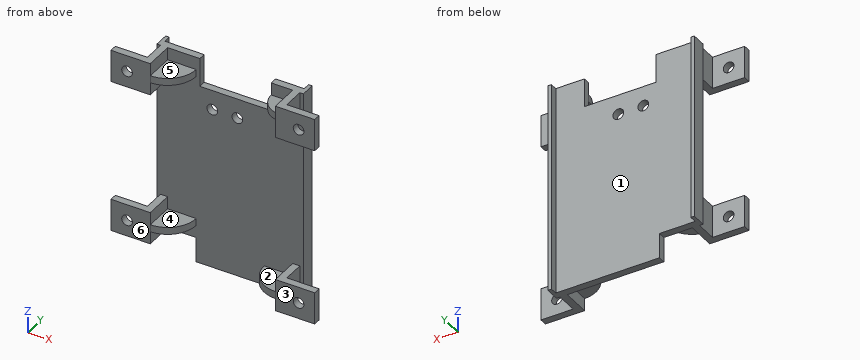
```python
from build123d import *

# Parameters (mm, degrees)
SKETCH1_W           = 57
SKETCH1_H           = 59
BOSS_EXTRUDE1_DEPTH = 10
SKETCH2_W           = 41
SKETCH2_H           = 10
CUT_EXTRUDE1_DEPTH  = 9
SKETCH4_W           = 10
SKETCH4_H           = 7
CUT_EXTRUDE3_DEPTH  = 83.643814046
SKETCH5_W           = 34
SKETCH5_H           = 10
CUT_EXTRUDE4_DEPTH  = 9
SKETCH8_W           = 20
SKETCH8_H           = 10
CUT_EXTRUDE5_DEPTH  = 8
SKETCH9_W           = 35
SKETCH9_H           = 59
CUT_EXTRUDE6_DEPTH  = 8
SKETCH10_W          = 9
SKETCH10_H          = 7
CUT_EXTRUDE7_DEPTH  = 83.643814046
SKETCH11_W          = 9
SKETCH11_H          = 9
CUT_EXTRUDE8_DEPTH  = 8
SKETCH12_W          = 9
SKETCH12_H          = 9
CUT_EXTRUDE9_DEPTH  = 8
SKETCH13_W          = 9
SKETCH13_H          = 9
CUT_EXTRUDE10_DEPTH = 8
SKETCH14_W          = 9
SKETCH14_H          = 9
CUT_EXTRUDE11_DEPTH = 8
SKETCH15_W          = 2
SKETCH15_H          = 41
CUT_EXTRUDE12_DEPTH = 8
SKETCH16_W          = 2
SKETCH16_H          = 34
CUT_EXTRUDE13_DEPTH = 8
SKETCH31_W          = 2
SKETCH31_H          = 8
REVOLVE3_ANGLE      = 90
SKETCH32_W          = 2
SKETCH32_H          = 8
REVOLVE4_ANGLE      = 90
SKETCH33_W          = 6
SKETCH33_H          = 2
REVOLVE5_ANGLE      = 90
SKETCH34_W          = 2
SKETCH34_H          = 8
REVOLVE6_ANGLE      = 90
SKETCH41_R          = 1.5
CUT_EXTRUDE14_DEPTH = 83.42572414
SKETCH42_R          = 1.5
CUT_EXTRUDE15_DEPTH = 83.643814046
SKETCH46_W          = 59
SKETCH46_H          = 2
BOSS_EXTRUDE3_DEPTH = 1
SKETCH47_W          = 1
SKETCH47_H          = 59
BOSS_EXTRUDE4_DEPTH = 2
SKETCH48_W          = 52
SKETCH48_H          = 2
BOSS_EXTRUDE5_DEPTH = 1
SKETCH49_W          = 1
SKETCH49_H          = 52
BOSS_EXTRUDE6_DEPTH = 2


with BuildPart() as part:
    # Sketch1 → Boss-Extrude1 (new body)
    with BuildSketch(Plane(origin=(0, 0, 0), x_dir=(1, 0, 0), z_dir=(0, 1, 0))):
        with Locations((28.5, 29.5)):
            Rectangle(SKETCH1_W, SKETCH1_H)
    extrude(amount=BOSS_EXTRUDE1_DEPTH)

    # Sketch2 → Cut-Extrude1 (cut)
    with BuildSketch(Plane(origin=(57, 0, 0), x_dir=(0, 0, -1), z_dir=(1, 0, 0))):
        with Locations((29.5, 5)):
            Rectangle(SKETCH2_W, SKETCH2_H)
    extrude(amount=-CUT_EXTRUDE1_DEPTH, mode=Mode.SUBTRACT)

    # Sketch4 → Cut-Extrude3 (cut, through all)
    with BuildSketch(Plane(origin=(0, 10, 0), x_dir=(1, 0, 0), z_dir=(0, 1, 0))):
        with Locations((5, 55.5)):
            Rectangle(SKETCH4_W, SKETCH4_H)
    extrude(amount=-CUT_EXTRUDE3_DEPTH, mode=Mode.SUBTRACT)

    # Sketch5 → Cut-Extrude4 (cut)
    with BuildSketch(Plane.ZY):
        with Locations((-26, 5)):
            Rectangle(SKETCH5_W, SKETCH5_H)
    extrude(amount=-CUT_EXTRUDE4_DEPTH, mode=Mode.SUBTRACT)

    # Sketch8 → Cut-Extrude5 (cut)
    with BuildSketch(Plane.XY):
        with Locations((30, 5)):
            Rectangle(SKETCH8_W, SKETCH8_H)
    extrude(amount=-CUT_EXTRUDE5_DEPTH, mode=Mode.SUBTRACT)

    # Sketch9 → Cut-Extrude6 (cut)
    with BuildSketch(Plane(origin=(0, 0, 0), x_dir=(-1, 0, 0), z_dir=(0, -1, 0))):
        with Locations((-28.5, 29.5)):
            Rectangle(SKETCH9_W, SKETCH9_H)
    extrude(amount=-CUT_EXTRUDE6_DEPTH, mode=Mode.SUBTRACT)

    # Sketch10 → Cut-Extrude7 (cut, through all)
    with BuildSketch(Plane(origin=(0, 10, 0), x_dir=(1, 0, 0), z_dir=(0, 1, 0))):
        with Locations((14.5, 55.5)):
            Rectangle(SKETCH10_W, SKETCH10_H)
    extrude(amount=-CUT_EXTRUDE7_DEPTH, mode=Mode.SUBTRACT)

    # Sketch11 → Cut-Extrude8 (cut)
    with BuildSketch(Plane(origin=(0, 10, 0), x_dir=(1, 0, 0), z_dir=(0, 1, 0))):
        with Locations((52.5, 4.5)):
            Rectangle(SKETCH11_W, SKETCH11_H)
    extrude(amount=-CUT_EXTRUDE8_DEPTH, mode=Mode.SUBTRACT)

    # Sketch12 → Cut-Extrude9 (cut)
    with BuildSketch(Plane(origin=(0, 10, 0), x_dir=(1, 0, 0), z_dir=(0, 1, 0))):
        with Locations((52.5, 54.5)):
            Rectangle(SKETCH12_W, SKETCH12_H)
    extrude(amount=-CUT_EXTRUDE9_DEPTH, mode=Mode.SUBTRACT)

    # Sketch13 → Cut-Extrude10 (cut)
    with BuildSketch(Plane(origin=(0, 10, 0), x_dir=(1, 0, 0), z_dir=(0, 1, 0))):
        with Locations((4.5, 47.5)):
            Rectangle(SKETCH13_W, SKETCH13_H)
    extrude(amount=-CUT_EXTRUDE10_DEPTH, mode=Mode.SUBTRACT)

    # Sketch14 → Cut-Extrude11 (cut)
    with BuildSketch(Plane(origin=(0, 10, 0), x_dir=(1, 0, 0), z_dir=(0, 1, 0))):
        with Locations((4.5, 4.5)):
            Rectangle(SKETCH14_W, SKETCH14_H)
    extrude(amount=-CUT_EXTRUDE11_DEPTH, mode=Mode.SUBTRACT)

    # Sketch15 → Cut-Extrude12 (cut)
    with BuildSketch(Plane(origin=(0, 0, 0), x_dir=(-1, 0, 0), z_dir=(0, -1, 0))):
        with Locations((-47, 29.5)):
            Rectangle(SKETCH15_W, SKETCH15_H)
    extrude(amount=-CUT_EXTRUDE12_DEPTH, mode=Mode.SUBTRACT)

    # Sketch16 → Cut-Extrude13 (cut)
    with BuildSketch(Plane(origin=(0, 0, 0), x_dir=(-1, 0, 0), z_dir=(0, -1, 0))):
        with Locations((-10, 26)):
            Rectangle(SKETCH16_W, SKETCH16_H)
    extrude(amount=-CUT_EXTRUDE13_DEPTH, mode=Mode.SUBTRACT)

    # Sketch31 → Revolve3 (revolve)
    with BuildSketch(Plane(origin=(11, 0, 0), x_dir=(0, 0, -1), z_dir=(1, 0, 0))):
        with Locations((4.5, 4)):
            Rectangle(SKETCH31_W, SKETCH31_H)
    revolve(axis=Axis((11, 8, -3.5), (0, 0, 1)), revolution_arc=REVOLVE3_ANGLE)

    # Sketch32 → Revolve4 (revolve)
    with BuildSketch(Plane(origin=(11, 0, 0), x_dir=(0, 0, -1), z_dir=(1, 0, 0))):
        with Locations((47.5, 4)):
            Rectangle(SKETCH32_W, SKETCH32_H)
    revolve(axis=Axis((11, 8, -46.5), (0, 0, 1)), revolution_arc=REVOLVE4_ANGLE)

    # Sketch33 → Revolve5 (revolve)
    with BuildSketch(Plane.XZ.offset(-8)):
        with Locations((43, -4.5)):
            Rectangle(SKETCH33_W, SKETCH33_H)
    revolve(axis=Axis((46, 8, -3.5), (0, 0, 1)), revolution_arc=REVOLVE5_ANGLE)

    # Sketch34 → Revolve6 (revolve)
    with BuildSketch(Plane.ZY.offset(-46)):
        with Locations((-54.5, 4)):
            Rectangle(SKETCH34_W, SKETCH34_H)
    revolve(axis=Axis((46, 8, -53.5), (0, 0, -1)), revolution_arc=REVOLVE6_ANGLE)

    # Sketch41 → Cut-Extrude14 (cut, through all)
    with BuildSketch(Plane(origin=(0, 2, 0), x_dir=(1, 0, 0), z_dir=(0, 1, 0))):
        with Locations(Location((52.5, 4.5, 0), (0, 0, 270))):
            Circle(SKETCH41_R)
        with Locations(Location((52.5, 54.5, 0), (0, 0, 270))):
            Circle(SKETCH41_R)
        with Locations(Location((4.5, 4.5, 0), (0, 0, 270))):
            Circle(SKETCH41_R)
        with Locations(Location((4.5, 47.5, 0), (0, 0, 270))):
            Circle(SKETCH41_R)
    extrude(amount=-CUT_EXTRUDE14_DEPTH, mode=Mode.SUBTRACT)

    # Sketch42 → Cut-Extrude15 (cut, through all)
    with BuildSketch(Plane(origin=(0, 10, 0), x_dir=(1, 0, 0), z_dir=(0, 1, 0))):
        with Locations(Location((23.5, 13.5, 0), (0, 0, 270))):
            Circle(SKETCH42_R)
        with Locations(Location((30.5, 13.5, 0), (0, 0, 270))):
            Circle(SKETCH42_R)
    extrude(amount=-CUT_EXTRUDE15_DEPTH, mode=Mode.SUBTRACT)

    # Sketch46 → Boss-Extrude3 (add)
    with BuildSketch(Plane(origin=(48, 0, 0), x_dir=(0, 0, -1), z_dir=(1, 0, 0))):
        with Locations((29.5, 9)):
            Rectangle(SKETCH46_W, SKETCH46_H)
    extrude(amount=BOSS_EXTRUDE3_DEPTH)

    # Sketch47 → Boss-Extrude4 (add)
    with BuildSketch(Plane(origin=(0, 10, 0), x_dir=(1, 0, 0), z_dir=(0, 1, 0))):
        with Locations((48.5, 29.5)):
            Rectangle(SKETCH47_W, SKETCH47_H)
    extrude(amount=BOSS_EXTRUDE4_DEPTH)

    # Sketch48 → Boss-Extrude5 (add)
    with BuildSketch(Plane.ZY.offset(-9)):
        with Locations((-26, 9)):
            Rectangle(SKETCH48_W, SKETCH48_H)
    extrude(amount=BOSS_EXTRUDE5_DEPTH)

    # Sketch49 → Boss-Extrude6 (add)
    with BuildSketch(Plane(origin=(0, 10, 0), x_dir=(1, 0, 0), z_dir=(0, 1, 0))):
        with Locations((8.5, 26)):
            Rectangle(SKETCH49_W, SKETCH49_H)
    extrude(amount=BOSS_EXTRUDE6_DEPTH)


solid = part.part
```
The model under review builds one solid part; all positions refer to its coordinate system, in mm. Face numbers are marked on the shaded views. A direction names the side the tool comes from. Round coordinates to 2 decimals unless told otherwise and drop trailing zeros. Order: outer loops, then holes, each group sorted by start corner. A loop starts at its lowest first (then second) coordinate and runs counter-clockwise, first axis right, second up. Notation, with made-up numbers: (63.25, 34.25) -> (97.25, 34.25) arc R23 cw to (97.25, 47.25) -> close; hole circle Ø9 at (13.5, 18). An arc over 180 degrees is marked (long way). Use a Markdown table: item, result.
Q1. For line 1 (Z direction, x = 44, y = 7.75); line 2 (Z direction, x = 17, y = 4.5); line 3 (X direction, y = 10.5, z = -41), list the stretches that pass through material, from the lowest coordinate up.
Values:
| item | result |
|---|---|
| line 1 | z = -55.5 to -53.5, -5.5 to -3.5 |
| line 2 | z = -48.5 to -46.5, -5.5 to -3.5 |
| line 3 | x = 8 to 9, 48 to 49 |
Q2. We need section B-B on x = 23.5. Write out the cut boundary in (y, z).
Values:
| item | result |
|---|---|
| outline | (8, -59) -> (10, -59) -> (10, -15) -> (8, -15) -> close; (8, -12) -> (10, -12) -> (10, -8) -> (8, -8) -> close |
Q3. We need section D-D on x = 4.5. Write out the cut boundary in (y, z), then the cut area to 3 significant figures.
Values:
| item | result |
|---|---|
| outline | (0, -52) -> (2, -52) -> (2, -49) -> (0, -49) -> close; (0, -46) -> (2, -46) -> (2, -43) -> (0, -43) -> close; (0, -9) -> (2, -9) -> (2, -6) -> (0, -6) -> close; (0, -3) -> (2, -3) -> (2, 0) -> (0, 0) -> close |
| area | 24.0 mm^2 |
Q4. We need section A-A on z = -4.5. State how many separate pieces and enclosed holes the cut face has, then the cut area to 3 significant figures.
Values:
| item | result |
|---|---|
| separate pieces | 4 |
| enclosed holes | 0 |
| area | 181 mm^2 |
Q5. We need section C-C on y = 11.25. Write out the cut boundary in (x, z), then the cut area to 3 significant figures.
Values:
| item | result |
|---|---|
| outline | (8, -52) -> (9, -52) -> (9, 0) -> (8, 0) -> close; (48, -59) -> (49, -59) -> (49, 0) -> (48, 0) -> close |
| area | 111 mm^2 |
Q6. Clearance check with flat-ended pins moving along their axes: P1, Ø7, axis at x = 3, z = -47, coming from the +Y side; P2, Ø6.5, axis at y = 5.5, z = -3, coming from the -X side; P3, Ø4, axis at x = 21, z = -42, coming from the -Y side. State where each tip first meets the part, or that it passes through.
Values:
| item | result |
|---|---|
| P1 | stops at y = 2 |
| P2 | stops at x = 8 |
| P3 | stops at y = 8 |
Q7. Tool access review of the marked faces 1, 2 and 3: name each direction out of +Z, -Z, +X, -X, +Y, -Y from which nothing blocks a thin tool from reaching the whole face with its end or side.
Values:
| item | result |
|---|---|
| face 1 | +Z, -Z, +Y |
| face 2 | -X, -Y |
| face 3 | +Z, -Z, +X, -X, -Y |
Q8. Mouldability with a two-part tool opening along Z and no side actions: class the marked faces 4, 5 and 6 as +Z half, -Z half, draft (parallel to the pull), parting line (faces both ways), or undercut.
Values:
| item | result |
|---|---|
| face 4 | undercut |
| face 5 | +Z half |
| face 6 | draft |
